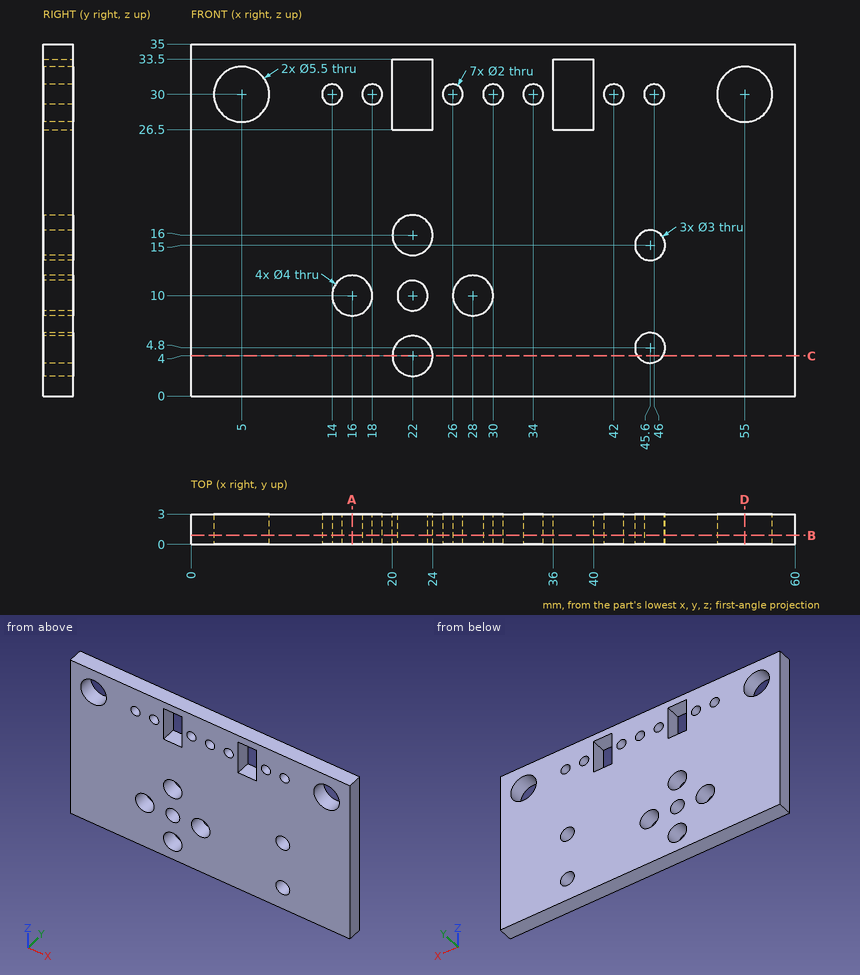
Source: three-view drawing plus pictorial views. Frame: mm from the lowest corner of the part. Round coordinates to 2 decimals unless told otherwise and drop trailing zeros. Loops run counter-clockwise (first coordinate to the right, second up) from the corner with the lowest first, then second, coordinate; pieces in that order, holes last.
Q1. Section D-D, the plane x = 55. Return loops of the section in (y, z).
Q2. Section B-B, the plane y = 0.9. State how many separate pieces and enclosed holes the cut face has, plus the area to 3 significant figures.
Q3. Section C-C, the plane z = 4. Return loops of the section in (x, y).
Q4. First-contact query: P1, Ø1.8, axis at x = 34, z = 30, coming from the -Y side. Flat tip, straight axial feed; report the tip coordinate or a pass-through.
Q5. Ray query, line 1 (Z direction, x = 22, y = 2.05); line 2 (Z direction, x = 45.6, y = 1.9); line 3 (Z direction, x = 5, y = 1.7). Return the intervals inside material, ascending.
Q6. Section A-A, the plane x = 16. Return loops of the section in (y, z), plus the area to 3 significant figures.
Solutions:
1. outline: (0, 0) - (3, 0) - (3, 27.25) - (0, 27.25) - close; (0, 32.75) - (3, 32.75) - (3, 35) - (0, 35) - close
2. separate pieces: 1
2. enclosed holes: 18
2. area: 1,900 mm2
3. outline: (0, 0) - (20, 0) - (20, 3) - (0, 3) - close; (24, 0) - (44.33, 0) - (44.33, 3) - (24, 3) - close; (46.87, 0) - (60, 0) - (60, 3) - (46.87, 3) - close
4. P1: passes through
5. line 1: z = 0 to 2, 6 to 8.5, 11.5 to 14, 18 to 26.5, 33.5 to 35
5. line 2: z = 0 to 3.3, 6.3 to 13.5, 16.5 to 29.08, 30.92 to 35
5. line 3: z = 0 to 27.25, 32.75 to 35
6. outline: (0, 0) - (3, 0) - (3, 8) - (0, 8) - close; (0, 12) - (3, 12) - (3, 35) - (0, 35) - close
6. area: 93.0 mm2
